Model file for the job. Use its own axes, mm. Face numbers are marked on the shaded views. Round coordinates to 2 decimals unless told otherwise and drop trailing zeros. Order: outer loops, then holes, each group sorted by start corner. A loop starts at its lowest first (then second) coordinate and runs counter-clockwise, first axis right, second up. Notation, with made-up numbers: (25.25, 5) - (61.25, 5) arc R22 ccw to (61.25, 26) - close; hole circle Ø4 at (15, -2). An arc over 180 degrees is marked (long way). Put each result on its own line as item: value. Start each with the question number.
Item 1: Saw through at C-C on z = 12. List the corners of the cut face in (x, y) (3 decimals), plus the area to 3 significant figures.
Item 2: Probe probe 1 along Y at (x, z) = (0, 8.3) (3 decimals); probe 2 along Y at (x, z) = (-1.35, 3.5); probe 3 along Z at (x, y) = (-0.8, -0.75). List the from-to ranges inside material, lowest first.
Item 3: Saw through at B-B on z = 6.5. List the corners of the cut face in (x, y) (3 decimals), plus the area to 3 significant figures.
Item 4: Saw through at A-A on x = 0. List the corners of the cut face in (y, z) (3 decimals).
Item 5: Pin check, flat tips, straight feed: pin 1 Ø1.2 at (x, y) = (-1, -0.5) entering from +Z; pin 2 Ø1 at (x, z) = (-2, 13.5) entering from +Y; pin 3 Ø1 at (y, z) = (-2, 7.5) entering from +X. Stop position of each tip, or through.
Item 6: Mould opens along Y. For the marked faces 1 and 2 say: pulls with the +Y half, pulls with the -Y half, needs draft (parallel to the pull), parting line crosses it, or undercut.
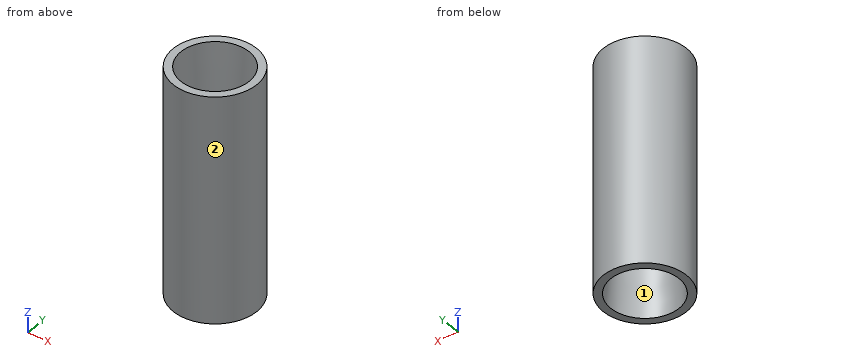
```python
from build123d import *

# Parameters (mm, degrees)
SKETCH1_R           = 2.775
BOSS_EXTRUDE1_DEPTH = 15
SKETCH2_R           = 2.27
CUT_EXTRUDE1_DEPTH  = 5.68
CUT_EXTRUDE1_TAPER  = 3.074
SKETCH7_R           = 1
CUT_EXTRUDE2_DEPTH  = 16
SKETCH9_R           = 2.27
CUT_EXTRUDE3_DEPTH  = 5.68
CUT_EXTRUDE3_TAPER  = 3.074


with BuildPart() as part:
    # Sketch1 → Boss-Extrude1 (new body)
    with BuildSketch(Plane.XY):
        Circle(SKETCH1_R)
    extrude(amount=BOSS_EXTRUDE1_DEPTH)

    # Sketch2 → Cut-Extrude1 (cut)
    with BuildSketch(Plane.XY):
        Circle(SKETCH2_R)
    extrude(amount=CUT_EXTRUDE1_DEPTH, taper=CUT_EXTRUDE1_TAPER, mode=Mode.SUBTRACT)

    # Sketch7 → Cut-Extrude2 (cut, through all)
    with BuildSketch(Plane.XY):
        Circle(SKETCH7_R)
    extrude(amount=CUT_EXTRUDE2_DEPTH, mode=Mode.SUBTRACT)

    # Sketch9 → Cut-Extrude3 (cut)
    with BuildSketch(Plane.XY.offset(15)):
        Circle(SKETCH9_R)
    extrude(amount=-CUT_EXTRUDE3_DEPTH, taper=CUT_EXTRUDE3_TAPER, mode=Mode.SUBTRACT)


solid = part.part
```
Results found:
1. outline: circle Ø5.55 at (0, 0); hole circle Ø4.218 at (0, 0)
1. area: 10.2 mm²
2. probe 1: y = -2.775 to -1, 1 to 2.775
2. probe 2: y = -2.42 to -1.59, 1.59 to 2.42
2. probe 3: z = 5.68 to 9.32
3. outline: circle Ø5.55 at (0, 0); hole circle Ø2 at (0, 0)
3. area: 21.1 mm²
4. outline: (-2.775, 0) - (-2.27, 0) - (-1.965, 5.68) - (-1, 5.68) - (-1, 9.32) - (-1.965, 9.32) - (-2.27, 15) - (-2.775, 15) - close; (1, 5.68) - (1.965, 5.68) - (2.27, 0) - (2.775, 0) - (2.775, 15) - (2.27, 15) - (1.965, 9.32) - (1, 9.32) - close
5. pin 1: stops at z = 9.32
5. pin 2: stops at y = 2.33
5. pin 3: stops at x = 2.33
6. face 1: undercut
6. face 2: parting line crosses it
